Can you work these out from the drawing? Everything is in mm from the part's minimum corner. Round coordinates to 2 decimals unless told otherwise and drop trailing zeros. Order: outer loops, then holes, each group sorted by start corner. A loop starts at its lowest first (then second) coordinate and runs counter-clockwise, first axis right, second up. Notation, with made-up numbers: (44, 68.5) -> (59, 68.5) arc R32 ccw to (59, 97.5) -> close; hole circle Ø8 at (-35, 54.5). An arc over 180 degrees is marked (long way). One line per item, written item: value.
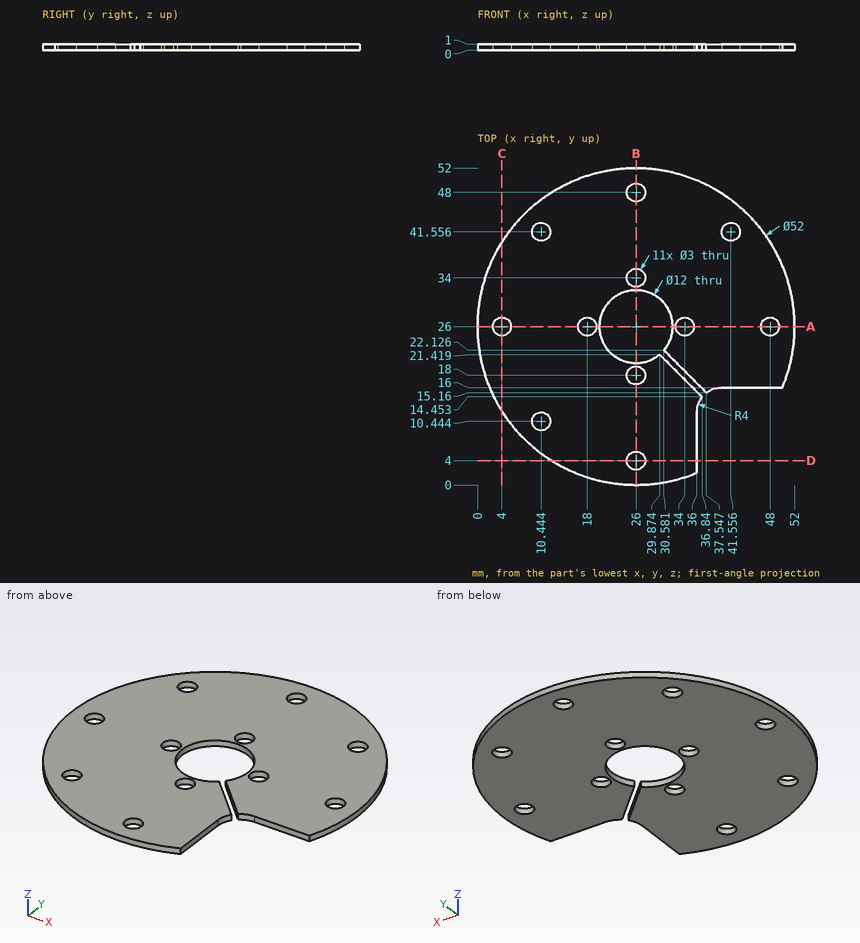
Q1. I want a section at C-C on x = 4. List the corners of the cut face in (y, z) for me.
Answers below:
outline: (12.14, 0) -> (24.5, 0) -> (24.5, 1) -> (12.14, 1) -> close; (27.5, 0) -> (39.86, 0) -> (39.86, 1) -> (27.5, 1) -> close
Q2. Will these pins go through, and if not, where does the flat tip stop? pin 1 Ø0.5 at (x, z) = (43.5, 0.5) entering from -Y; pin 2 Ø0.5 at (y, z) = (9.5, 0.5) entering from +X.
Answers below:
pin 1: y = 16
pin 2: x = 36
Q3. I want a section at A-A on y = 26. List the corners of the cut face in (x, z) for me.
Answers below:
outline: (0, 0) -> (2.5, 0) -> (2.5, 1) -> (0, 1) -> close; (5.5, 0) -> (16.5, 0) -> (16.5, 1) -> (5.5, 1) -> close; (19.5, 0) -> (20, 0) -> (20, 1) -> (19.5, 1) -> close; (32, 0) -> (32.5, 0) -> (32.5, 1) -> (32, 1) -> close; (35.5, 0) -> (46.5, 0) -> (46.5, 1) -> (35.5, 1) -> close; (49.5, 0) -> (52, 0) -> (52, 1) -> (49.5, 1) -> close
Q4. Please list where these lines run through material, in increasing order: line 1 along Y through (x, z) = (26, 0.75); line 2 along Y through (x, z) = (27, 0.7) (1 decimal).
Answers below:
line 1: 0 to 2.5, 5.5 to 16.5, 19.5 to 20, 32 to 32.5, 35.5 to 46.5, 49.5 to 52
line 2: 0 to 2.9, 5.1 to 16.9, 19.1 to 20.1, 31.9 to 32.9, 35.1 to 46.9, 49.1 to 52
Q5. I want a section at D-D on y = 4. List the corners of the cut face in (x, z) for me.
Answers below:
outline: (12.14, 0) -> (24.5, 0) -> (24.5, 1) -> (12.14, 1) -> close; (27.5, 0) -> (36, 0) -> (36, 1) -> (27.5, 1) -> close
